Autodesk Inventor part; units mm, degrees
ref_plane "YZ Plane" through (0, 0, 0) normal (1, 0, 0) x (0, 1, 0)
ref_plane "XZ Plane" through (0, 0, 0) normal (0, 1, 0) x (-1, 0, 0)
ref_plane "XY Plane" through (0, 0, 0) normal (0, 0, 1) x (1, 0, 0)
sketch "Sketch1" plane through (0, 0, 0) normal (0, 1, 0) x (-1, 0, 0)
  line L0 (176.8421, 47.7193) -> (-23.1579, 47.7193)
  line L1 (-23.1579, 47.7193) -> (-23.1579, -52.2807)
  line L2 (-23.1579, -52.2807) -> (176.8421, -52.2807)
  line L3 (176.8421, -52.2807) -> (176.8421, 47.7193)
  point P0 (0, 0)
  dimension "d0" = 100
  dimension "d1" = 200
extrude "Extrusion1" add sketch "Sketch1" along normal blind 15
fillet "Fillet2" radius 60 1 edges at (-176.8421, 7.5, -52.2807)
sketch "Sketch2" plane through (0, 15, 0) normal (0, 1, 0) x (1, 0, 0)
  arc A0 (-116.8421, 52.2807) -> (-176.8421, -7.7193) centre (-116.8421, -7.7193) ccw
  circle A1 centre (-116.8421, -7.7193) radius 11.1579
  point P0 (0, 0)
extrude "Extrusion2" cut sketch "Sketch2" against normal blind 15
properties part number "PovorotBlockOsnova"
Geometry: final body of the model. Coordinates: model frame, mm. Round coordinates to 2 decimals unless told otherwise and drop trailing zeros. Loops run counter-clockwise (first coordinate to the right, second up) from the corner with the lowest first, then second, coordinate; pieces in that order, holes last. Notation, with made-up numbers: M 44,65.25 L 100,65.25 A16 ccw 100,96.25 Z; hole C 45,-25.75 d7. An arc over 180 degrees is marked long. One line per question, with ' | ' between items.
(1) Material intervals for line 1 along Z through (x, y) = (-108, 12.75); line 2 along Z through (x, y) = (-108.5, 5.25); line 3 along X through (y, z) = (7.75, -45), sorted ascending. Write a range as from..to.
Check result:
line 1: z = -52.28..0.91, 14.52..47.72 | line 2: z = -52.28..0.31, 15.13..47.72 | line 3: x = -145.49..23.16
(2) Contact query for flat-ended pins moving along their axis: P1, Ø1.5, axis at x = -112.5, z = -12, coming from the -Y side; P2, Ø1.5, axis at y = 13.5, z = -10.5, coming from the -X side. Output: stop coordinate, or through.
Check result:
P1: stops at y = 0 | P2: stops at x = -174.24
(3) Cut plane D-D on z = -22. Return the cut outline in (x, y).
Check result:
outline: M -168.96,0 L 23.16,0 L 23.16,15 L -168.96,15 Z
(4) Cut plane A-A on y = 4. Return the cut outline in (x, z), plus the area to 3 significant figures.
Check result:
outline: M -176.84,7.72 A60 ccw -116.84,-52.28 L 23.16,-52.28 L 23.16,47.72 L -176.84,47.72 Z; hole C -116.84,7.72 d22.32 | area: 18,800 mm2
(5) Pull-direction query (X, two-part tool) for faces 1 (the cylindrical face through (-158.8, 7.6, -35.17)), 2 (the cylindrical face through (-127.99, 7.6, 7.23)), 3 (the flat face through (-75, 15, -2)); classes: +X half, -X half, draft (parallel to the pull), parting line (faces both ways), or undercut.
Check result:
face 1: -X half | face 2: undercut | face 3: draft
(6) Cut plane C-C on x = -148.5. Return the cut outline in (y, z).
Check result:
outline: M 0,-43.25 L 15,-43.25 L 15,47.72 L 0,47.72 Z
(7) Cut plane B-B on z = 4. Return the cut outline in (x, y), plus the area to 3 significant figures.
Check result:
outline: M -176.73,0 L -127.36,0 L -127.36,15 L -176.73,15 Z; M -106.32,0 L 23.16,0 L 23.16,15 L -106.32,15 Z | area: 2,680 mm2
